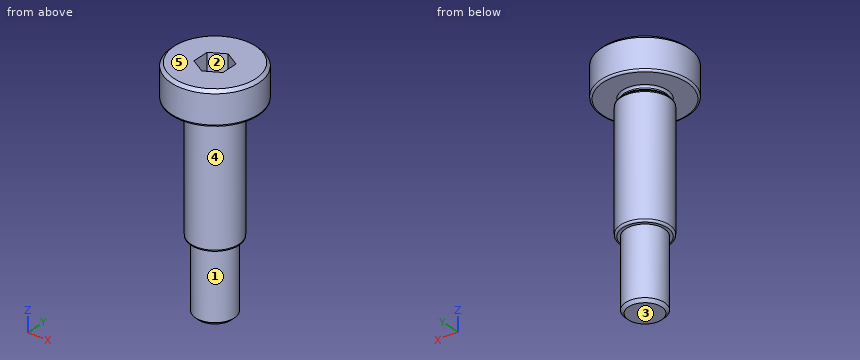
Solid Edge part; units mm, degrees
sketch "Sketch1" plane through (0, 0, 0) normal (0, -1, 0) x (1, 0, 0)
  line L0 (0, 23.7) -> (4.505, 23.7)
  line L1 (4.505, 23.7) -> (4.505, 20.25)
  line L2 (4.505, 20.25) -> (2.1, 20.25)
  line L3 (2.1, 20.25) -> (2.1, 19.85)
  line L4 (2.1, 19.85) -> (2.5, 19.85)
  line L5 (2.5, 19.85) -> (2.5, 7.25)
  line L6 (2.5, 7.25) -> (2, 7.25)
  line L7 (2, 7.25) -> (2, 0)
  line L8 (2, 0) -> (0, 0)
  dimension "D1" = 4.505
  dimension "D2" = 2.1
  dimension "D3" = 2
  dimension "D4" = 2.5
  dimension "D5" = 2
revolve "RevolvedProtrusion1" add sketch "Sketch1" angle 360 about axis through (0, 0, 0) along (0, 0, 1)
chamfer "Chamfer1" distance 0.3 angle 45 3 edges at (-2.5, 0, 19.85) (-4.505, 0, 23.7) (-2, 0, 0)
fillet "Round_1" radius 0.2 4 edges at (-4.505, 0, 20.25) (-2.1, 0, 20.25) (-2.5, 0, 7.25) (-2.5, 0, 19.55)
sketch "Sketch2" plane through (0, 0, 23.7) normal (0, 0, 1) x (1, 0, 0)
  line L0 (1.5, 0.866) -> (0, 1.7321)
  line L1 (0, 1.7321) -> (-1.5, 0.866)
  line L2 (-1.5, 0.866) -> (-1.5, -0.866)
  line L3 (-1.5, -0.866) -> (0, -1.7321)
  line L4 (0, -1.7321) -> (1.5, -0.866)
  line L5 (1.5, -0.866) -> (1.5, 0.866)
extrude "ExtrudedCutout_1" cut sketch "Sketch2" against normal blind 2.4
properties material "Stainless Steel, 304"
Work out the finished part from the listing and answer in its coordinate system (mm). Face numbers are marked on the shaded views. A direction names the side the tool comes from. Round coordinates to 2 decimals unless told otherwise and drop trailing zeros. Order: outer loops, then holes, each group sorted by start corner. A loop starts at its lowest first (then second) coordinate and runs counter-clockwise, first axis right, second up.
Q1. Find the intervals of material crossed by line 1 along Z through (x, y) = (-3, -0.75); line 2 along X through (y, z) = (1.5, 22.5); line 3 along Y through (x, z) = (2, 19.25), in increasing order.
Solution:
line 1: z = 20.25 to 23.7
line 2: x = -4.25 to -0.4, 0.4 to 4.25
line 3: y = -1.5 to 1.5
Q2. A tool of negligible diameter and unlimited length cuts with its end or side. For the marked faces 4 and 5, from which of +Z, -Z, +X, -X, +Y, -Y can it reach the whole face along a straight path? Write none if from no direction.
Solution:
face 4: -Z
face 5: +Z, +X, -X, +Y, -Y
Q3. The mould has two halves that part along Y. Classify the marked faces 1, 2 and 3: pulls with the +Y half, pulls with the -Y half, needs draft (parallel to the pull), parting line crosses it, or undercut.
Solution:
face 1: parting line crosses it
face 2: undercut
face 3: needs draft
Q4. Given pin 1 Ø1 at (x, z) = (-2.5, 18.5) entering from +Y; pin 2 Ø1.3 at (x, y) = (-0.5, 0) entering from +Z; pin 3 Ø4.5 at (x, y) = (0, 1) entering from -Z; pin 4 Ø4 at (y, z) = (-2.5, 11) entering from +X, each flat-ended and moving along its own axis, determine where each tip first touches the part or whether it passes through.
Solution:
pin 1: stops at y = 1.5
pin 2: stops at z = 21.3
pin 3: stops at z = 0
pin 4: stops at x = 2.45
Q5. A cutting plane is placed at A-A, the plane z = 14. Determine the outline of the cut face in (x, y).
Solution:
outline: circle Ø5 at (0, 0)
